Design review of the part built by this model. Coordinates are the model's own, in mm. Face numbers are marked on the shaded views. A direction names the side the tool comes from. Coordinates: 2 decimals unless noted, no trailing zeros. Write each loop counter-clockwise with the first axis right and the second up, starting at its lowest first coordinate (ties: lowest second). Pieces come first, ordered by that corner, then holes.
Q1. Take a section at C-C (x = -320). Give the boundary of the cut face in (y, z) (3 decimals), and give its area (3 significant figures).
Q2. Insertion check: pin 1 (3 mm diameter, centred on y = 5, z = 12.5, fed in from -X); pin 2 (12 mm diameter, centred on x = -107, y = 17, fed in from +Z) (3 decimals); pin 3 (11 mm diameter, centred on x = -211.5, z = 15, fed in from +Y) (3 decimals). Each pin has a flat end and moves straight along its axis. Give the tip position at first contact, or say it passes through.
Q3. Take a section at A-A (x = -101.6). Give the boundary of the cut face in (y, z) (1 decimal), and give its area (3 significant figures).
Q4. Machinability: for the marked faces 1 and 2, which of the approach directions +Z, -Z, +X, -X, +Y, -Y give a long, thin tool a straight path to every point of the face, cutting with its end or side? Answer none if there is none.
Q5. For probe 1 along Z at (x, y) = (-101.6, 1.4); probe 2 along X at (y, z) = (1.75, 12.25) (3 decimals); probe 3 along Y at (x, z) = (-138, 15) (3 decimals), list the stretches that pass through material, from the lowest coordinate up.
Q6. Take a section at B-B (y = 19.25). Give the boundary of the cut face in (x, z) (3 decimals), and give its area (3 significant figures).
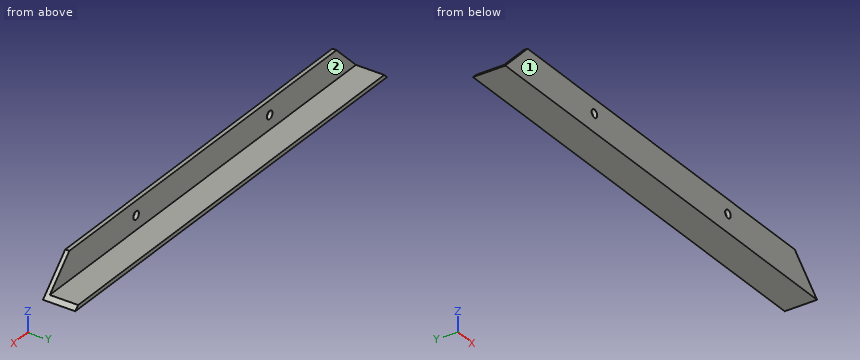
```python
from build123d import *

# Parameters (mm, degrees)
SKETCH2_W           = 355.6
SKETCH2_H           = 25.4
BOSS_EXTRUDE1_DEPTH = 3.175
SKETCH3_W           = 355.6
SKETCH3_H           = 3.175
BOSS_EXTRUDE2_DEPTH = 22.225
CUT_EXTRUDE3_DEPTH  = 25.4
SKETCH7_R           = 3.175
CUT_EXTRUDE4_DEPTH  = 3.175


with BuildPart() as part:
    # Sketch2 → Boss-Extrude1 (new body)
    with BuildSketch(Plane(origin=(0, 0, 0), x_dir=(1, 0, 0), z_dir=(0, 1, 0))):
        with Locations((-177.8, -12.7)):
            Rectangle(SKETCH2_W, SKETCH2_H)
    extrude(amount=BOSS_EXTRUDE1_DEPTH)

    # Sketch3 → Boss-Extrude2 (add)
    with BuildSketch(Plane(origin=(0, 3.175, 0), x_dir=(1, 0, 0), z_dir=(0, 1, 0))):
        with Locations((-177.8, -1.5875)):
            Rectangle(SKETCH3_W, SKETCH3_H)
    extrude(amount=BOSS_EXTRUDE2_DEPTH)

    # Sketch6 → Cut-Extrude3 (cut)
    with BuildSketch(Plane(origin=(0, 25.4, 0), x_dir=(1, 0, 0), z_dir=(0, 1, 0))):
        Polygon((-355.6, 0), (-314.465679006, -41.134320994), (-387.836085875, -49.332490233), align=None)
        Polygon((0, 0), (-41.658764664, -41.658764664), (40.75579897, -53.520309566), align=None)
    extrude(amount=-CUT_EXTRUDE3_DEPTH, mode=Mode.SUBTRACT)

    # Sketch7 → Cut-Extrude4 (cut)
    with BuildSketch(Plane(origin=(0, 3.175, 0), x_dir=(1, 0, 0), z_dir=(0, 1, 0))):
        with Locations((-101.6, -14.2875)):
            Circle(SKETCH7_R)
        with Locations((-254, -14.2875)):
            Circle(SKETCH7_R)
    extrude(amount=-CUT_EXTRUDE4_DEPTH, mode=Mode.SUBTRACT)


solid = part.part
```
Response:
1. outline: (0, 0) - (25.4, 0) - (25.4, 3.175) - (3.175, 3.175) - (3.175, 25.4) - (0, 25.4) - close
1. area: 151 mm2
2. pin 1: passes through
2. pin 2: stops at z = 3.175
2. pin 3: stops at y = 3.175
3. outline: (0, 0) - (25.4, 0) - (25.4, 3.2) - (3.2, 3.2) - (3.2, 11.1) - (0, 11.1) - close; (0, 17.5) - (3.2, 17.5) - (3.2, 25.4) - (0, 25.4) - close
3. area: 131 mm2
4. face 1: +Z, -Z, +X, -X, -Y
4. face 2: +Z, +X, -X, +Y
5. probe 1: z = 0 to 11.11, 17.46 to 25.4
5. probe 2: x = -343.35 to -256.435, -251.565 to -104.035, -99.165 to -12.25
5. probe 3: y = 0 to 3.175
6. outline: (-355.6, 0) - (0, 0) - (-3.175, 3.175) - (-352.425, 3.175) - close
6. area: 1,120 mm2
